Model file for the job. Use its own axes, mm. Round coordinates to 2 decimals unless told otherwise and drop trailing zeros. Order: outer loops, then holes, each group sorted by start corner. A loop starts at its lowest first (then second) coordinate and runs counter-clockwise, first axis right, second up. Notation, with made-up numbers: (54, 35.5) - (78, 35.5) arc R15 cw to (78, 64.5) - close; hole circle Ø1 at (18.25, 62). An arc over 180 degrees is marked (long way). Use one line per item in the form item = value.
from build123d import *

# Parameters (mm, degrees)
SKETCH1_R               = 12.7
BOSS_EXTRUDE1_DEPTH     = 6.35
CUT_EXTRUDE1_DEPTH      = 20.05
CUT_EXTRUDE1_DEPTH_BACK = 20.05
SKETCH2_R               = 1.7359375


with BuildPart() as part:
    # Sketch1 → Boss-Extrude1 (new body)
    # profile 1 of 2: a face of its own
    with BuildSketch(Plane.XY):
        Circle(SKETCH1_R)
        with BuildLine():
            ThreePointArc((2.2225, 2.267403526), (-3.175, 0), (2.2225, -2.267403526))
            Line((2.2225, -2.267403526), (2.2225, 2.267403526))
        make_face(mode=Mode.SUBTRACT)
    # profile 2 of 2: a face of its own
    with BuildSketch(Plane.XY):
        with BuildLine():
            Line((2.2225, 2.267403526), (2.2225, -2.267403526))
            ThreePointArc((2.2225, -2.267403526), (-3.175, 0), (2.2225, 2.267403526))
        make_face()
        with BuildLine():
            ThreePointArc((2.1225, 2.224998596), (-3.075, 0), (2.1225, -2.224998596))
            Line((2.1225, -2.224998596), (2.1225, 2.224998596))
        make_face(mode=Mode.SUBTRACT)
    extrude(amount=BOSS_EXTRUDE1_DEPTH)

    # Sketch2 → Cut-Extrude1 (cut, two sides: drawn at the far end of the back side and taken through both)
    with BuildSketch(Plane.XY.offset(6.35).offset(-CUT_EXTRUDE1_DEPTH_BACK)):
        with Locations((7.9375, 0)):
            Circle(SKETCH2_R)
        with Locations((-7.9375, 0)):
            Circle(SKETCH2_R)
    extrude(amount=CUT_EXTRUDE1_DEPTH + CUT_EXTRUDE1_DEPTH_BACK, mode=Mode.SUBTRACT)


solid = part.part
(1) Slice it at B-B on y = 0. Count the separate pieces of the cut face and the enclosed holes in it, then the cut area to 3 significant figures.
Report:
separate_pieces = 4
enclosed_holes = 0
area = 84.2 mm2
(2) Pin check, flat tips, straight feed: pin 1 (3 mm diameter, centred on x = 4.5, z = 4, fed in from -Y); pin 2 (1.5 mm diameter, centred on x = -9.5, z = 2, fed in from -Y); pin 3 (1 mm diameter, centred on x = 1.5, z = 3.5, fed in from +Y). Stop position of each tip, or through.
Report:
pin_1 = -12.34
pin_2 = -9.2
pin_3 = 12.66
(3) Slice it at D-D on x = 7.5. Give the cut face in (y, z).
Report:
outline = (-10.25, 0) - (-1.68, 0) - (-1.68, 6.35) - (-10.25, 6.35) - close; (1.68, 0) - (10.25, 0) - (10.25, 6.35) - (1.68, 6.35) - close
(4) Probe probe 1 along Y at (x, z) = (0, 3.25) (3 decimals); probe 2 along X at (y, z) = (-1.5, 1); probe 3 along X at (y, z) = (-2.25, 2). List the from-to ranges inside material, lowest first. Write a range as [from, to].
Report:
probe_1 = [-12.7, -3.075], [3.075, 12.7]
probe_2 = [-12.61, -8.81], [-7.06, -2.68], [2.12, 7.06], [8.81, 12.61]
probe_3 = [-12.5, -2.1], [2.1, 12.5]
(5) Pull direction Y, two halves, no side cores. Call faces 1 (the face through (-2.75, -12.4, 3.13)), 2 (the face through (2.122, 0, 3)), 3 (the face through (3, 0, 0)): released by +Y, released by -Y, zero draft, split by the parting line, or undercut.
Report:
face_1 = split by the parting line
face_2 = undercut
face_3 = zero draft
(6) Slice it at A-A on x = 0. Give the cut face in (y, z) (3 decimals), then the cut area to 3 significant figures.
Report:
outline = (-12.7, 0) - (-3.075, 0) - (-3.075, 6.35) - (-12.7, 6.35) - close; (3.075, 0) - (12.7, 0) - (12.7, 6.35) - (3.075, 6.35) - close
area = 122 mm2
